Geometry: see drawing. Coordinates: mm, zero at the bounding-box minimum. A direction names the side the tool comes from. Give positions to 0.01 mm unless a question says otherwise; leave off trailing zeros. Write each loop counter-clockwise with the first axis right and the second up, starting at its lowest first coordinate (ties: lowest second). Pieces come first, ordered by that corner, then holes. Notation, with made-up numbers: (-38.75, 22.25) - (-16.75, 22.25) arc R34 cw to (-16.75, 52.25) - close; hole circle Ø4 at (84.5, -33.75). An arc over 180 degrees is marked (long way). Return JSON: item names as keys, results as strings.
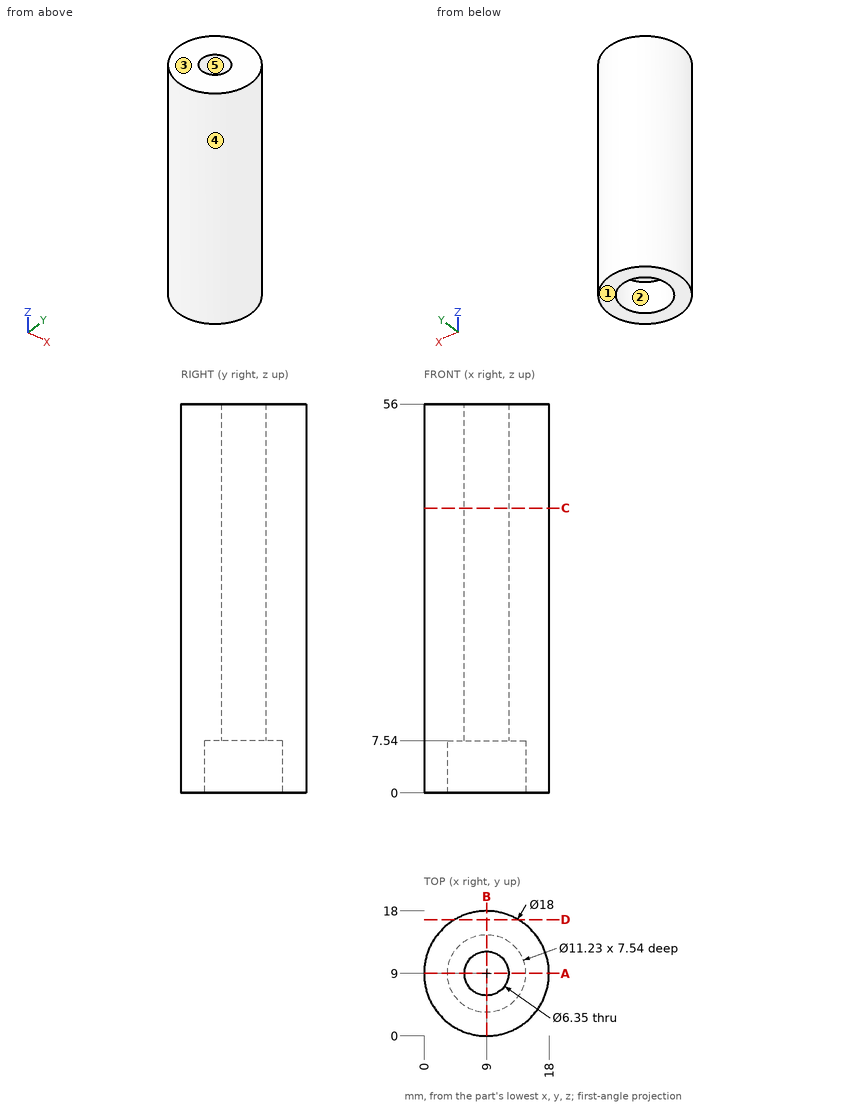
Q1. Section query D-D, the plane y = 16.75. Return the cut outline in (x, z), plus the area to 3 significant figures.
Answer key:
{"outline": "(4.42, 0) - (13.58, 0) - (13.58, 56) - (4.42, 56) - close", "area": "512 mm^2"}
Q2. Set-up query: the marked faces 1 and 2. Return all of +Z, -Z, +X, -X, +Y, -Y with unobstructed straight access to the full face (end or side cutting, diameter ignored); none if empty.
Answer key:
{"face 1": "-Z, +X, -X, +Y, -Y", "face 2": "-Z"}
Q3. Section query A-A, the plane y = 9. Return the cut outline in (x, z) (3 decimals).
Answer key:
{"outline": "(0, 0) - (3.385, 0) - (3.385, 7.54) - (5.825, 7.54) - (5.825, 56) - (0, 56) - close; (12.175, 7.54) - (14.615, 7.54) - (14.615, 0) - (18, 0) - (18, 56) - (12.175, 56) - close"}
Q4. Material intervals for probe 1 along Y at (x, z) = (9, 48) (3 decimals); probe 2 along Y at (x, z) = (9, 5.25) (3 decimals); probe 3 along Z at (x, y) = (8.75, 5.5), sorted ascending. Write a range as [from, to].
Answer key:
{"probe 1": "y = [0, 5.825], [12.175, 18]", "probe 2": "y = [0, 3.385], [14.615, 18]", "probe 3": "z = [7.54, 56]"}
Q5. Pin query (flat end, axial travel): P1, Ø5, axis at x = 4.5, z = 11, coming from the -Y side; P2, Ø5, axis at y = 12, z = 40.5, coming from the +X side; P3, Ø1.5, axis at x = 10.5, z = 18, coming from the -Y side. Return the tip coordinate at first contact, or that it passes through.
Answer key:
{"P1": "stops at y = 0.23", "P2": "stops at x = 17.99", "P3": "stops at y = 0.03"}
Q6. Section query C-C, the plane z = 41. Return the cut outline in (x, y) (3 decimals), plus the area to 3 significant figures.
Answer key:
{"outline": "circle Ø18 at (9, 9); hole circle Ø6.35 at (9, 9)", "area": "223 mm^2"}
Q7. Mould query, pull axis X, two halves, no side actions, for the marked faces 3, 4 and 5. Classes: pulls with the +X half, pulls with the -X half, needs draft (parallel to the pull), parting line crosses it, or undercut.
Answer key:
{"face 3": "needs draft", "face 4": "parting line crosses it", "face 5": "undercut"}
